```python
from build123d import *

# Parameters (mm, degrees)
BATTERY_BASE_DEPTH = 36.5
PINS_DEPTH         = 6.5


with BuildPart() as part:
    # Battery Base Sketch → Battery Base (new body)
    with BuildSketch(Plane.XY):
        with BuildLine():
            Line((-10.775, 4.725), (10.775, 4.725))
            ThreePointArc((10.775, 4.725), (15.5, 0), (10.775, -4.725))
            Line((10.775, -4.725), (-10.775, -4.725))
            ThreePointArc((-10.775, -4.725), (-15.5, 0), (-10.775, 4.725))
        make_face()
    extrude(amount=BATTERY_BASE_DEPTH)

    # Pins Sketch → Pins (cut)
    with BuildSketch(Plane(origin=(0, 0, 0), x_dir=(-1, 0, 0), z_dir=(0, 0, -1))):
        with BuildLine():
            Line((-15.499933862, -0.025), (15.499933862, -0.025))
            ThreePointArc((15.499933862, -0.025), (14.124906715, 3.332228984), (10.775, 4.725))
            Line((10.775, 4.725), (-10.775, 4.725))
            ThreePointArc((-10.775, 4.725), (-14.124906715, 3.332228984), (-15.499933862, -0.025))
        make_face()
    extrude(amount=-PINS_DEPTH, mode=Mode.SUBTRACT)


solid = part.part
```
Geometry: final body of the model. Coordinates: model frame, mm. A direction names the side the tool comes from. Coordinates: 2 decimals unless noted, no trailing zeros. Order: outer loops, then holes, each group sorted by start corner. A loop starts at its lowest first (then second) coordinate and runs counter-clockwise, first axis right, second up. Notation, with made-up numbers: M 50,-36 L 80,-36 A30 cw 80,-9 Z; hole C 45.25,-27.75 d5. An arc over 180 degrees is marked long. Answer in a Markdown table with one row per item. Add a question column.
Q1. Section query A-A on x = -8. Return the cut outline in (y, z) (3 decimals), and give its area (3 significant figures).
Q2. Section query D-D on x = -11.5. Return the cut outline in (y, z) (3 decimals), and give its area (3 significant figures).
Q3. Section query C-C on y = -2.75. Return the cut outline in (x, z), and give its area (3 significant figures).
Q4. Contact query for a flat-ended pin moving along its axis: P1, Ø2, axis at x = 5, y = 3, coming from the -Z side. Output: stop coordinate, or through.
Q5. Reachability of faces 1 (the flat face through (0, -4.725, 18)), 2 (the flat face through (0, 2, 6.5)) from +Z, -Z, +X, -X, +Y, -Y: full face, straight path, thin tool, end or side. Return the list, or none.
Q6. Line query: L1, parallel to Z at x = 2.5, y = 1; L2, parallel to Y at x = 0.5, z = 5 (3 decimals); L3, parallel to X at y = -0.25, z = 19.5. Output: solid intervals per line, ascending.
Q7. Section query B-B on z = 3.5. Return the cut outline in (x, y) (3 decimals).
Completed:
| question | item | result |
|---|---|---|
| 1 | outline | M -4.725,0 L -0.025,0 L -0.025,6.5 L 4.725,6.5 L 4.725,36.5 L -4.725,36.5 Z |
| 1 | area | 314 mm2 |
| 2 | outline | M -4.669,0 L -0.025,0 L -0.025,6.5 L 4.669,6.5 L 4.669,36.5 L -4.669,36.5 Z |
| 2 | area | 310 mm2 |
| 3 | outline | M -14.62,0 L 14.62,0 L 14.62,36.5 L -14.62,36.5 Z |
| 3 | area | 1,070 mm2 |
| 4 | P1 | stops at z = 6.5 |
| 5 | face 1 | +Z, -Z, +X, -X, -Y |
| 5 | face 2 | -Z, +X, -X, +Y |
| 6 | L1 | z = 6.5 to 36.5 |
| 6 | L2 | y = -4.725 to -0.025 |
| 6 | L3 | x = -15.49 to 15.49 |
| 7 | outline | M -15.5,-0.025 A4.725 ccw -10.775,-4.725 L 10.775,-4.725 A4.725 ccw 15.5,-0.025 Z |
